The drawing under review shows one solid part. Ordinate dimensions are in mm from its lowest x, y, z. Give positions to 0.01 mm unless a question says otherwise; leave off trailing zeros. Write each loop counter-clockwise with the first axis right and the second up, starting at its lowest first coordinate (ties: lowest second). Pieces come first, ordered by that corner, then holes.
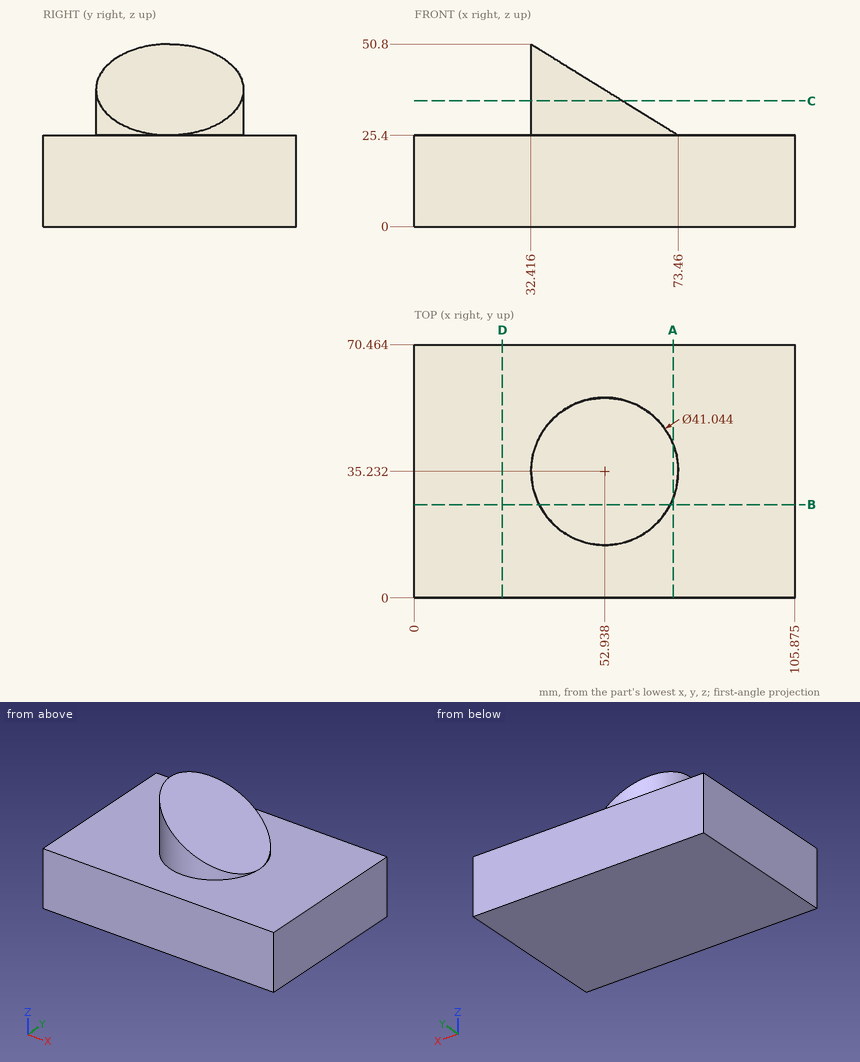
1) Consider section C-C, the plane z = 35. Give the boundary of the cut face in (x, y).
2) To check wall thickness, follow probe 1 along Z at (x, y) = (21.5, 7); probe 2 along Y at (x, z) = (44.5, 41.5) (1 decimal); probe 3 along Z at (x, y) = (52, 42). State the ranges of each line that lie inside material, in increasing order.
3) Insertion check: pin 1 (6 mm diameter, centred on y = 40.5, z = 37, fed in from +X) (1 decimal); pin 2 (10 mm diameter, centred on y = 37.5, z = 36.5, fed in from -X); pin 3 (12 mm diameter, centred on x = 84, y = 34.5, fed in from +Z). Each pin has a flat end and moves straight along its axis. Give the tip position at first contact, or say it passes through.
4) Consider section A-A, the plane x = 72. Give the boundary of the cut face in (y, z) (1 decimal).
5) Consider section B-B, the plane y = 26. Give the boundary of the cut face in (x, z) (1 decimal).
6) Consider section D-D, the plane x = 24.5. Give the boundary of the cut face in (y, z) (1 decimal), then the cut area to 3 significant figures.
Answer block:
1. outline: (57.95, 15.33) - (57.95, 55.13) arc R20.52 ccw (long way) to start
2. probe 1: z = 0 to 25.4
2. probe 2: y = 16.5 to 53.9
2. probe 3: z = 0 to 38.68
3. pin 1: stops at x = 59.6
3. pin 2: stops at x = 32.42
3. pin 3: stops at z = 25.4
4. outline: (0, 0) - (70.5, 0) - (70.5, 25.4) - (42.8, 25.4) - (42.8, 26.3) - (27.6, 26.3) - (27.6, 25.4) - (0, 25.4) - close
5. outline: (0, 0) - (105.9, 0) - (105.9, 25.4) - (71.3, 25.4) - (71.3, 26.8) - (34.6, 49.4) - (34.6, 25.4) - (0, 25.4) - close
6. outline: (0, 0) - (70.5, 0) - (70.5, 25.4) - (0, 25.4) - close
6. area: 1,790 mm2
